```python
from build123d import *

# Parameters (mm, degrees)
PAD_DEPTH        = 1
POCKET_DEPTH     = 0.001
HOLE_D           = 1.75
HOLE_CSINK_D     = 3.3
HOLE_CSINK_ANGLE = 90
SKETCH023_R      = 4.9
HOLE014_DEPTH    = 25
SKETCH024_R      = 1.5
HOLE015_DEPTH    = 25
SKETCH025_R      = 5.25
SKETCH025_R_2    = 1.5
POCKET007_DEPTH  = 5


with BuildPart() as part:
    # Sketch → Pad (new body)
    with BuildSketch(Plane.XY):
        with BuildLine():
            Line((-51.8, 52.175), (51.8, 52.175))
            ThreePointArc((52.175, 51.8), (52.065165, 52.065165), (51.8, 52.175))
            Line((52.175, 51.8), (52.175, -51.8))
            ThreePointArc((51.8, -52.175), (52.065165, -52.065165), (52.175, -51.8))
            Line((51.8, -52.175), (-51.8, -52.175))
            ThreePointArc((-52.175, -51.8), (-52.065165, -52.065165), (-51.8, -52.175))
            Line((-52.175, -51.8), (-52.175, 51.8))
            ThreePointArc((-51.8, 52.175), (-52.065165, 52.065165), (-52.175, 51.8))
        make_face()
    extrude(amount=-PAD_DEPTH)

    # Sketch002 → Pocket (cut, through all)
    with BuildSketch(Plane.XY.offset(-4.8)):
        with BuildLine():
            Line((-45, 50.175), (45, 50.175))
            ThreePointArc((45, 50.175), (45.353553, 50.321447), (45.5, 50.675))
            ThreePointArc((45.5, 50.675), (45.353553, 51.028553), (45, 51.175))
            Line((-45, 51.175), (45, 51.175))
            ThreePointArc((-45, 51.175), (-45.353553, 51.028553), (-45.5, 50.675))
            ThreePointArc((-45.5, 50.675), (-45.353553, 50.321447), (-45, 50.175))
        make_face()
        with BuildLine():
            Line((-45, -51.175), (45, -51.175))
            ThreePointArc((45, -51.175), (45.353553, -51.028553), (45.5, -50.675))
            ThreePointArc((45.5, -50.675), (45.353553, -50.321447), (45, -50.175))
            Line((-45, -50.175), (45, -50.175))
            ThreePointArc((-45, -50.175), (-45.353553, -50.321447), (-45.5, -50.675))
            ThreePointArc((-45.5, -50.675), (-45.353553, -51.028553), (-45, -51.175))
        make_face()
        with BuildLine():
            Line((51.175, -45), (51.175, 45))
            ThreePointArc((51.175, 45), (51.028553, 45.353553), (50.675, 45.5))
            ThreePointArc((50.675, 45.5), (50.321447, 45.353553), (50.175, 45))
            Line((50.175, -45), (50.175, 45))
            ThreePointArc((50.175, -45), (50.321447, -45.353553), (50.675, -45.5))
            ThreePointArc((50.675, -45.5), (51.028553, -45.353553), (51.175, -45))
        make_face()
        with BuildLine():
            Line((-50.175, -45), (-50.175, 45))
            ThreePointArc((-50.175, 45), (-50.321447, 45.353553), (-50.675, 45.5))
            ThreePointArc((-50.675, 45.5), (-51.028553, 45.353553), (-51.175, 45))
            Line((-51.175, -45), (-51.175, 45))
            ThreePointArc((-51.175, -45), (-51.028553, -45.353553), (-50.675, -45.5))
            ThreePointArc((-50.675, -45.5), (-50.321447, -45.353553), (-50.175, -45))
        make_face()
    extrude(amount=-POCKET_DEPTH, mode=Mode.SUBTRACT)

    # Hole (through all)
    with Locations(Plane.XY):
        with Locations((-50, 50), (50, 50), (50, -50), (-50, -50)):
            CounterSinkHole(HOLE_D / 2, HOLE_CSINK_D / 2, counter_sink_angle=HOLE_CSINK_ANGLE)

    # Sketch023 → Hole014 (cut)
    with BuildSketch(Plane.XY):
        with Locations((-40.005, -13.335)):
            Circle(SKETCH023_R)
        with Locations((-13.335, -13.335)):
            Circle(SKETCH023_R)
        with Locations((13.335, -13.335)):
            Circle(SKETCH023_R)
        with Locations((40.005, -13.335)):
            Circle(SKETCH023_R)
        with Locations((-40.005, -40.005)):
            Circle(SKETCH023_R)
        with Locations((-13.335, -40.005)):
            Circle(SKETCH023_R)
        with Locations((13.335, -40.005)):
            Circle(SKETCH023_R)
        with Locations((40.005, -40.005)):
            Circle(SKETCH023_R)
    extrude(amount=-HOLE014_DEPTH, mode=Mode.SUBTRACT)

    # Sketch024 → Hole015 (cut)
    with BuildSketch(Plane.XY):
        with Locations((-40.005, -4.835)):
            Circle(SKETCH024_R)
        with Locations((-13.335, -4.835)):
            Circle(SKETCH024_R)
        with Locations((13.335, -4.835)):
            Circle(SKETCH024_R)
        with Locations((40.005, -4.835)):
            Circle(SKETCH024_R)
        with Locations((-40.005, -31.505)):
            Circle(SKETCH024_R)
        with Locations((-13.335, -31.505)):
            Circle(SKETCH024_R)
        with Locations((13.335, -31.505)):
            Circle(SKETCH024_R)
        with Locations((40.005, -31.505)):
            Circle(SKETCH024_R)
    extrude(amount=-HOLE015_DEPTH, mode=Mode.SUBTRACT)

    # Sketch025 → Pocket007 (cut)
    with BuildSketch(Plane.XY):
        with Locations((-26.67, 26.67)):
            Circle(SKETCH025_R)
        with Locations((26.67, 26.67)):
            Circle(SKETCH025_R)
        with Locations((-47.515079, 36.39022)):
            Circle(SKETCH025_R_2)
        with Locations((-45.510497, 39.862258)):
            Circle(SKETCH025_R_2)
        with Locations((-42.933456, 42.933456)):
            Circle(SKETCH025_R_2)
        with Locations((-39.862258, 45.510497)):
            Circle(SKETCH025_R_2)
        with Locations((-36.39022, 47.515079)):
            Circle(SKETCH025_R_2)
        with Locations((5.824921, 36.39022)):
            Circle(SKETCH025_R_2)
        with Locations((7.829503, 39.862258)):
            Circle(SKETCH025_R_2)
        with Locations((10.406544, 42.933456)):
            Circle(SKETCH025_R_2)
        with Locations((13.477742, 45.510497)):
            Circle(SKETCH025_R_2)
        with Locations((16.94978, 47.515079)):
            Circle(SKETCH025_R_2)
    extrude(amount=-POCKET007_DEPTH, mode=Mode.SUBTRACT)


solid = part.part
```
Geometry: final body of the model. Coordinates: model frame, mm. Give positions to 0.01 mm unless a question says otherwise; leave off trailing zeros. Write each loop counter-clockwise with the first axis right and the second up, starting at its lowest first coordinate (ties: lowest second). Pieces come first, ordered by that corner, then holes.
1. Section query B-B, the plane x = 40. Return loops of the section in (y, z) (3 decimals), then the cut area to 4 significant figures.
2. Section query A-A, the plane y = 26.67. Return loops of the section in (x, z) (3 decimals).
3. Pin query (flat end, axial travel): P1, Ø15.5, axis at x = 40.005, y = -40.005, coming from the +Z side; P2, Ø6.5, axis at x = -26.67, y = 26.67, coming from the +Z side; P3, Ø2.5, axis at x = 50, y = -50, coming from the +Z side. Return the tip coordinate at first contact, or that it passes through.
4. Section query D-D, the plane z = -0.6. Count the separate pieces of the cut face and the enclosed holes in it, then the cut area to 3 significant figures.
5. Draft query along X for faces 1 (the flat face through (1, 1, 0)), 2 (the cylindrical face through (44.53, -15.21, -0.49)). Return one class per face: released by +X, released by -X, zero draft, split by the parting line, or undercut.
6. Line query: probe 1 along Y at (x, z) = (-14.5, -0.6) (1 decimal); probe 2 along Y at (x, z) = (39, -0.5) (3 decimals); probe 3 along Y at (x, z) = (17.5, -0.7) (3 decimals). Output: solid intervals per line, ascending.
7. Section query C-C, the plane x = 26.67. Return loops of the section in (y, z) (3 decimals), then the cut area to 4 significant figures.
Computed:
1. outline: (-52.175, -1) - (-44.905, -1) - (-44.905, 0) - (-52.175, 0) - close; (-35.105, -1) - (-33.005, -1) - (-33.005, 0) - (-35.105, 0) - close; (-30.005, -1) - (-18.235, -1) - (-18.235, 0) - (-30.005, 0) - close; (-8.435, -1) - (-6.335, -1) - (-6.335, 0) - (-8.435, 0) - close; (-3.335, -1) - (52.175, -1) - (52.175, 0) - (-3.335, 0) - close
1. area: 78.75 mm2
2. outline: (-52.175, -1) - (-31.92, -1) - (-31.92, 0) - (-52.175, 0) - close; (-21.42, -1) - (21.42, -1) - (21.42, 0) - (-21.42, 0) - close; (31.92, -1) - (52.175, -1) - (52.175, 0) - (31.92, 0) - close
3. P1: stops at z = 0
3. P2: passes through
3. P3: stops at z = -0.4
4. separate pieces: 1
4. enclosed holes: 32
4. area: 9,970 mm2
5. face 1: zero draft
5. face 2: undercut
6. probe 1: y = -52.2 to -44.8, -35.2 to -32.4, -30.6 to -18.1, -8.6 to -5.8, -3.9 to 52.2
6. probe 2: y = -52.175 to -44.801, -35.209 to -32.619, -30.391 to -18.131, -8.539 to -5.949, -3.721 to 52.175
6. probe 3: y = -52.175 to -42.586, -37.424 to -15.916, -10.754 to 46.12, 48.911 to 52.175
7. outline: (-52.175, -1) - (21.42, -1) - (21.42, 0) - (-52.175, 0) - close; (31.92, -1) - (52.175, -1) - (52.175, 0) - (31.92, 0) - close
7. area: 93.85 mm2
